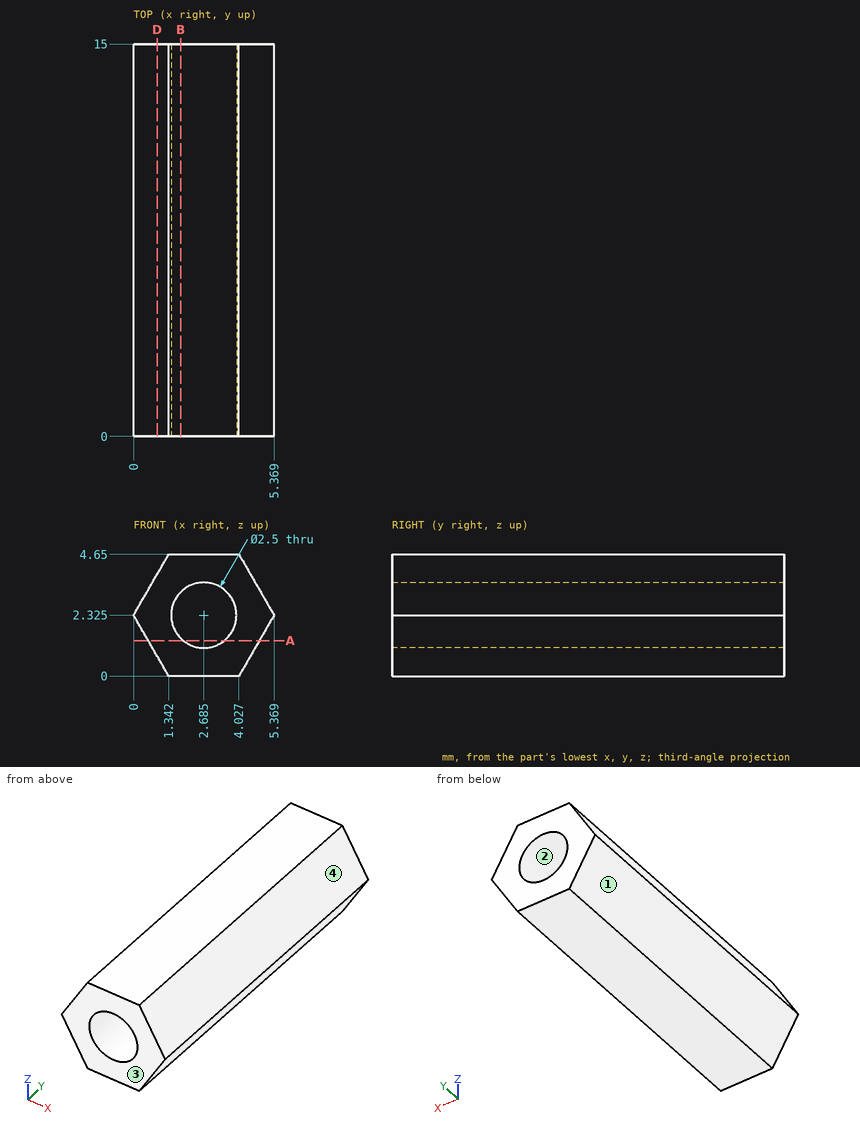
The figure shows three views and two pictorial views of one solid part (mm, origin at its lowest corner). Answer the questions. Give positions to 0.01 mm unless a question says otherwise; leave off trailing zeros. Order: outer loops, then holes, each group sorted by start corner. A loop starts at its lowest first (then second) coordinate and runs counter-clockwise, first axis right, second up. Notation, with made-up numbers: M 38,72 L 79,72 A30 ccw 79,95 Z; hole C 23.25,74.5 d5. An arc over 180 degrees is marked long. Return JSON: item names as keys, results as strings.
Q1. Find section D-D, the plane x = 0.9. Write down the section's boundary in (y, z).
Answer below:
{"outline": "M 0,0.77 L 15,0.77 L 15,3.88 L 0,3.88 Z"}
Q2. Find the intervals of material crossed by line 1 along Z through (x, y) = (2.1, 5.5); line 2 along X through (y, z) = (1.5, 1.7); line 3 along X through (y, z) = (12.25, 2.15), in increasing order. Write a range as [from, to].
Answer below:
{"line 1": "z = [0, 1.22], [3.43, 4.65]", "line 2": "x = [0.36, 1.6], [3.77, 5.01]", "line 3": "x = [0.1, 1.45], [3.92, 5.27]"}
Q3. The mould has two halves that part along X. Classify the marked faces 1, 2, 3 and 4: pulls with the +X half, pulls with the -X half, needs draft (parallel to the pull), parting line crosses it, or undercut.
Answer below:
{"face 1": "pulls with the -X half", "face 2": "undercut", "face 3": "needs draft", "face 4": "pulls with the +X half"}
Q4. Each of these flat-tipped pins is pushed along its axis until it touches: pin 1 (3 mm diameter, centred on x = 4, y = 12, fed in from -Z); pin 2 (1.5 mm diameter, centred on x = 0.5, y = 7.5, fed in from -Z). Where does it stop, or does it pass through?
Answer below:
{"pin 1": "stops at z = 0", "pin 2": "stops at z = 0.16"}
Q5. Find section A-A, the plane z = 1.35. Write down the section's boundary in (x, y).
Answer below:
{"outline": "M 0.56,0 L 1.9,0 L 1.9,15 L 0.56,15 Z; M 3.47,0 L 4.81,0 L 4.81,15 L 3.47,15 Z"}
Q6. Find section B-B, the plane x = 1.8. Write down the section's boundary in (y, z).
Answer below:
{"outline": "M 0,0 L 15,0 L 15,1.44 L 0,1.44 Z; M 0,3.21 L 15,3.21 L 15,4.65 L 0,4.65 Z"}
